Input: part model. Units: mm. Frame: model coordinates. Face numbers are marked on the shaded views. A direction names the side the tool comes from. Coordinates: 2 decimals unless noted, no trailing zeros. Loops run counter-clockwise (first coordinate to the right, second up) from the corner with the lowest first, then second, coordinate; pieces in that order, holes last.
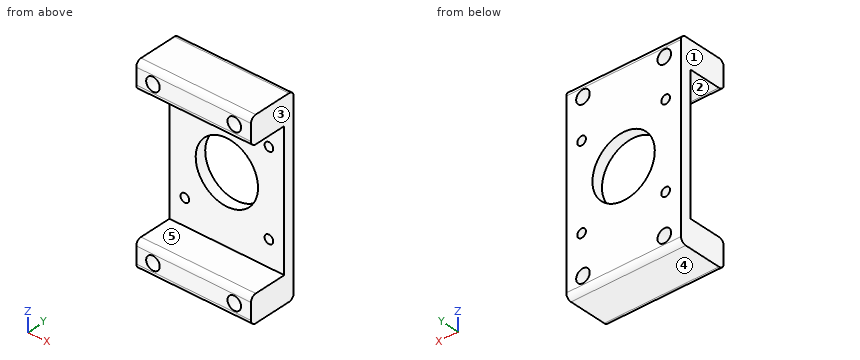
```python
from build123d import *

# Parameters (mm, degrees)
ESBO_O1_W                 = 50
ESBO_O1_H                 = 4
RESSALTO_EXTRUS_O1_DEPTH  = 21.15
ESBO_O3_R                 = 11.5
CORTE_EXTRUS_O1_DEPTH     = 45.680224932
ESBO_O4_R                 = 1.6
CORTE_EXTRUS_O2_DEPTH     = 45.680224932
PADR_OCIRCULAR1_COUNT     = 4
ESBO_O5_R                 = 2.5
CORTE_EXTRUS_O3_DEPTH     = 45.680224932
ESPELHAR2_COPY_1_SKETCH_R = 2.5
ESPELHAR2_COPY_1_DEPTH    = 45.680224932
FILETE1_R                 = 2


with BuildPart() as part:
    # Esboço1 → Ressalto-extrusão1 (new, symmetric)
    with BuildSketch(Plane(origin=(0, 0, 0), x_dir=(0, 0, -1), z_dir=(1, 0, 0))):
        Polygon((-25, -2), (-25, 2), (-35, 2), (-35, -16), (-25, -16), align=None)
        Rectangle(ESBO_O1_W, ESBO_O1_H)
        Polygon((35, 2), (25, 2), (25, -2), (25, -16), (35, -16), align=None)
    extrude(amount=RESSALTO_EXTRUS_O1_DEPTH, both=True)

    # Esboço3 → Corte-extrusão1 (cut, through all)
    with BuildSketch(Plane(origin=(0, 2, 0), x_dir=(1, 0, 0), z_dir=(0, 1, 0))):
        with Locations(Location((0, 0, 0), (0, 0, 270))):
            Circle(ESBO_O3_R)
    extrude(amount=-CORTE_EXTRUS_O1_DEPTH, mode=Mode.SUBTRACT)

    # Esboço4 → Corte-extrusão2 (cut, through all)
    with BuildSketch(Plane(origin=(0, 2, 0), x_dir=(1, 0, 0), z_dir=(0, 1, 0))):
        with Locations(Location((-15.5, 15.5, 0), (0, 0, 270))):
            Circle(ESBO_O4_R)
    corte_extrus_o2 = extrude(amount=-CORTE_EXTRUS_O2_DEPTH, mode=Mode.SUBTRACT)

    # PadrãoCircular1: Corte-extrusão2 ×4 about axis
    padr_ocircular1_axis = Axis((0, 0, 0), (0, 1, 0))
    for i in range(1, PADR_OCIRCULAR1_COUNT):
        add(corte_extrus_o2.rotate(padr_ocircular1_axis, i * 360 / PADR_OCIRCULAR1_COUNT), mode=Mode.SUBTRACT)

    # Esboço5 → Corte-extrusão3 (cut, through all)
    with BuildSketch(Plane.XZ.offset(16)):
        with Locations(Location((15, -30, 0), (0, 0, 270))):
            Circle(ESBO_O5_R)
    corte_extrus_o3 = extrude(amount=-CORTE_EXTRUS_O3_DEPTH, mode=Mode.SUBTRACT)

    # Espelhar1: Corte-extrusão3 across plane
    add(corte_extrus_o3.mirror(Plane(origin=(0, 0, 0), x_dir=(0, 0, 1), z_dir=(1, 0, 0))), mode=Mode.SUBTRACT)

    # Espelhar2: Corte-extrusão3 across plane
    add(corte_extrus_o3.mirror(Plane.XY), mode=Mode.SUBTRACT)

    # Espelhar2 copy 1 sketch → Espelhar2 copy 1 (cut, through all)
    with BuildSketch(Plane(origin=(0, -16, 0), x_dir=(-1, 0, 0), z_dir=(0, -1, 0))):
        with Locations(Location((15, -30, 0), (0, 0, 270))):
            Circle(ESPELHAR2_COPY_1_SKETCH_R)
    extrude(amount=-ESPELHAR2_COPY_1_DEPTH, mode=Mode.SUBTRACT)

    # Filete1
    filete1_edges = [part.edges().sort_by_distance(p)[0] for p in [
        (0, 2, -35),
        (0, -16, -35),
        (0, -16, -25),
        (0, -16, 25),
        (0, -16, 35),
        (0, 2, 35),
    ]]
    fillet(filete1_edges, radius=FILETE1_R)


solid = part.part
```
Item 1: Section query B-B (z = -15.5). Output: boundary loops of the cut face in (x, y), then the cut area to 3 significant figures.
Result:
outline: (-21.15, -2) - (-17.1, -2) - (-17.1, 2) - (-21.15, 2) - close; (-13.9, -2) - (13.9, -2) - (13.9, 2) - (-13.9, 2) - close; (17.1, -2) - (21.15, -2) - (21.15, 2) - (17.1, 2) - close
area: 144 mm2
Item 2: Section query D-D (x = -19). Output: boundary loops of the cut face in (y, z).
Result:
outline: (-16, -33) arc R2 ccw to (-14, -35) - (0, -35) arc R2 ccw to (2, -33) - (2, 33) arc R2 ccw to (0, 35) - (-14, 35) arc R2 ccw to (-16, 33) - (-16, 27) arc R2 ccw to (-14, 25) - (-2, 25) - (-2, -25) - (-14, -25) arc R2 ccw to (-16, -27) - close
Item 3: Mould query, pull axis Z, two halves, no side actions, for the marked faces 3, 4 and 5. Classes: +Z half, -Z half, draft (parallel to the pull), parting line (faces both ways), or undercut.
Result:
face 3: draft
face 4: -Z half
face 5: undercut
Item 4: Section query C-C (x = 0). Output: boundary loops of the cut face in (y, z).
Result:
outline: (-16, -33) arc R2 ccw to (-14, -35) - (0, -35) arc R2 ccw to (2, -33) - (2, -11.5) - (-2, -11.5) - (-2, -25) - (-14, -25) arc R2 ccw to (-16, -27) - close; (-16, 27) arc R2 ccw to (-14, 25) - (-2, 25) - (-2, 11.5) - (2, 11.5) - (2, 33) arc R2 ccw to (0, 35) - (-14, 35) arc R2 ccw to (-16, 33) - close
Item 5: Line query: L1, parallel to X at y = -8, z = -30; L2, parallel to Z at x = 16.5, y = -14.75; L3, parallel to Z at x = 15.5, y = 1.1. Output: solid intervals per line, ascending.
Result:
L1: x = -21.15 to -17.5, -12.5 to 12.5, 17.5 to 21.15
L2: z = -34.85 to -32, -28 to -25.15, 25.15 to 28, 32 to 34.85
L3: z = -34.67 to -32.45, -27.55 to -17.1, -13.9 to 13.9, 17.1 to 27.55, 32.45 to 34.67
Item 6: Reachability of the marked faces 1 and 2 from +Z, -Z, +X, -X, +Y, -Y: full face, straight path, thin tool, end or side. Return the list, or none.
Result:
face 1: +Z, -Z, -X, +Y, -Y
face 2: +X, -X, -Y
Item 7: Section query A-A (y = -4.5). Output: boundary loops of the cut face in (x, z).
Result:
outline: (-21.15, -35) - (21.15, -35) - (21.15, -25) - (-21.15, -25) - close; (-21.15, 25) - (21.15, 25) - (21.15, 35) - (-21.15, 35) - close; hole circle Ø5 at (-15, -30); hole circle Ø5 at (-15, 30); hole circle Ø5 at (15, -30); hole circle Ø5 at (15, 30)
Item 8: Contact query for flat-ended pins moving along their axis: P1, Ø21, axis at x = -1, z = -1.5, coming from the -Y side; P2, Ø14, axis at x = 0, z = 0, coming from the -Y side. Output: stop coordinate, or through.
Result:
P1: stops at y = -2
P2: passes through
